from build123d import *

# Parameters (mm, degrees)
SKETCH4_R           = 3.96875
BOSS_EXTRUDE1_DEPTH = 17.5895
SKETCH5_W           = 32.258
SKETCH5_H           = 32.3469
CUT_EXTRUDE1_DEPTH  = 149.479
CUT_EXTRUDE2_REACH  = 129.277
CUT_EXTRUDE3_REACH  = 126.564
SKETCH8_R           = 4.19735
BOSS_EXTRUDE2_DEPTH = 5.4102
SKETCH9_R           = 14.8209
CUT_EXTRUDE4_DEPTH  = 102.6


with BuildPart() as part:
    # Sketch3 → Revolve1 (revolve)
    with BuildSketch(Plane.XY):
        with BuildLine():
            Line((0, 0), (22.1742, 0))
            Line((22.1742, 0), (22.1742, 6.7818))
            ThreePointArc((22.1742, 6.7818), (21.430251224, 8.577851224), (19.6342, 9.3218))
            Line((19.6342, 9.3218), (18.3134, 9.3218))
            Line((18.3134, 9.3218), (18.3134, 97.6884))
            Line((18.3134, 97.6884), (19.431, 97.6884))
            ThreePointArc((19.431, 97.6884), (21.227051224, 98.432348776), (21.971, 100.2284))
            Line((21.971, 100.2284), (21.971, 101.6))
            Line((21.971, 101.6), (0, 101.6))
            Line((0, 101.6), (0, 0))
        make_face()
    revolve(axis=Axis((0, 101.6, 0), (0, -1, 0)))

    # Sketch4 → Boss-Extrude1 (add, symmetric)
    with BuildSketch(Plane(origin=(0, 0, 0), x_dir=(0, 0, -1), z_dir=(1, 0, 0))):
        Polygon((3.319704812, 97.6884), (115.572791881, -37.744541555), (116.058945734, -61.655625383), (109.136154682, -67.393554854), (97.331039415, -71.002358659), (0, 46.427186637), align=None)
        with Locations((105.157137902, -57.289139694)):
            Circle(SKETCH4_R, mode=Mode.SUBTRACT)
    extrude(amount=BOSS_EXTRUDE1_DEPTH, both=True)

    # Sketch5 → Cut-Extrude1 (cut)
    with BuildSketch(Plane(origin=(0, -93.569618845, -77.554828616), x_dir=(1, 0, 0), z_dir=(0, -0.769917596, -0.638143319))):
        with Locations((0, -47.261148993)):
            Rectangle(SKETCH5_W, SKETCH5_H)
    extrude(amount=-CUT_EXTRUDE1_DEPTH, mode=Mode.SUBTRACT)

    # Sketch6 → Cut-Extrude2 (cut, up to next)
    with BuildSketch(Plane(origin=(0, 41.412373886, -49.963878576), x_dir=(-1, 0, 0), z_dir=(0, 0.638143319, -0.769917596)), mode=Mode.PRIVATE) as cut_extrude2_sk1:
        with BuildLine():
            Line((14.9225, -97.744891724), (14.9225, -112.907394914))
            Line((14.9225, -112.907394914), (-14.9225, -112.907394914))
            Line((-14.9225, -112.907394914), (-14.9225, -97.744891724))
            ThreePointArc((-14.9225, -97.744891724), (0, -82.822391724), (14.9225, -97.744891724))
        make_face()
    cut_extrude2_tool1 = extrude(cut_extrude2_sk1.sketch, amount=-CUT_EXTRUDE2_REACH, mode=Mode.PRIVATE) & part.part
    add(cut_extrude2_tool1.solids().sort_by_distance((0, -35.009466, -113.305835))[0], mode=Mode.SUBTRACT)

    # Sketch7 → Cut-Extrude3 (cut, up to next)
    with BuildSketch(Plane(origin=(0, 18.906399111, -22.81050181), x_dir=(1, 0, 0), z_dir=(0, -0.638143319, 0.769917596)), mode=Mode.PRIVATE) as cut_extrude3_sk1:
        with BuildLine():
            Line((-9.989016296, -117.386717047), (9.989016296, -117.386717047))
            ThreePointArc((9.989016296, -117.386717047), (0, -106.76951783), (-9.989016296, -117.386717047))
        make_face()
    cut_extrude3_tool1 = extrude(cut_extrude3_sk1.sketch, amount=-CUT_EXTRUDE3_REACH, mode=Mode.PRIVATE) & part.part
    add(cut_extrude3_tool1.solids().sort_by_distance((0, -67.984352, -94.829576))[0], mode=Mode.SUBTRACT)

    # Sketch8 → Boss-Extrude2 (add)
    with BuildSketch(Plane(origin=(17.5895, 0, 0), x_dir=(0, 0, -1), z_dir=(1, 0, 0))):
        with Locations((81.207034429, -28.363574673)):
            Circle(SKETCH8_R)
    boss_extrude2 = extrude(amount=BOSS_EXTRUDE2_DEPTH)

    # Mirror1: Boss-Extrude2 across plane
    add(boss_extrude2.mirror(Plane(origin=(0, 0, 0), x_dir=(0, 0, 1), z_dir=(1, 0, 0))))

    # Sketch9 → Cut-Extrude4 (cut, through all)
    with BuildSketch(Plane.XZ):
        Circle(SKETCH9_R)
    extrude(amount=-CUT_EXTRUDE4_DEPTH, mode=Mode.SUBTRACT)


solid = part.part
The listing builds one solid part. Answer for the finished solid, in the listing's coordinates (mm). A direction names the side the tool comes from. Give positions to 0.01 mm unless a question says otherwise; leave off trailing zeros. Write each loop counter-clockwise with the first axis right and the second up, starting at its lowest first coordinate (ties: lowest second). Pieces come first, ordered by that corner, then holes. Notation, with made-up numbers: (-10, 2) - (34, 2) arc R25 cw to (34, 15) - close; hole circle Ø1 at (2, 35.25). An arc over 180 degrees is marked (long way). One line per question, with ' | ' between items. Start each with the question number.
1. Given P1, Ø6, axis at x = 12.5, z = -86.5, coming from the +Y side; P2, Ø23.5, axis at x = 0, z = 0, coming from the +Y side; P3, Ø13.5, axis at x = -3.5, z = -10, coming from the -Y side; P4, Ø12, axis at x = -0.5, z = -34.5, coming from the +Y side, each flat-ended and moving along its own axis, determine where each tip first touches the part or whether it passes through.
2. Section C-C, the plane x = 0 is taken. Count the separate pieces of the cut face and the enclosed holes in it, then the cut area to 3 significant figures.
3. Section A-A, the plane z = 0 is taken. Determine the outline of the cut face in (x, y).
4. Straight lines are drawn through the part: line 1 (X direction, y = 46, z = -37); line 2 (Z direction, x = -9.5, y = 52); line 3 (Y direction, x = -13.5, z = -59.5). For each, find the intervals that lie inside material, in ascending order.
5. For faces 4 (the face through (-17.6, 3.44, -13.49)), 5 (the face through (-20.26, -30.92, -77.88)), 6 (the face through (-18, 9.322, -6)), determine the directions among +Z, -Z, +X, -X, +Y, -Y from which every point of the face is accessible in a straight line to the end or side of a thin tool.
6. Section D-D, the plane y = 35 is taken. Determine the outline of the cut face in (x, z), then the cut area to 3 significant figures.
7. Determine the mould class of faces 1 (the face through (14.922, -36.4, -113.5)), 2 (the face through (-16.305, -69.724, -101.512)), 3 (the face through (16.129, -7, -67)) for opening direction Z: +Z half, -Z half, draft (parallel to the pull), parting line (faces both ways), or undercut.
8. Section B-B, the plane y = 17.5 is taken. Determine the outline of the cut face in (x, z), then the cut area to 3 significant figures.
Result:
1) P1: stops at y = 0.95 | P2: passes through | P3: stops at y = 0 | P4: stops at y = 67.31
2) separate pieces: 3 | enclosed holes: 0 | area: 1,250 mm2
3) outline: (-22.17, 0) - (-14.82, 0) - (-14.82, 101.6) - (-21.97, 101.6) - (-21.97, 100.23) arc R2.54 ccw to (-19.43, 97.69) - (-18.31, 97.69) - (-18.31, 9.32) - (-19.63, 9.32) arc R2.54 ccw to (-22.17, 6.78) - close; (14.82, 0) - (22.17, 0) - (22.17, 6.78) arc R2.54 ccw to (19.63, 9.32) - (18.31, 9.32) - (18.31, 97.69) - (19.43, 97.69) arc R2.54 ccw to (21.97, 100.23) - (21.97, 101.6) - (14.82, 101.6) - close
4) line 1: x = -17.59 to -16.13, 16.13 to 17.59 | line 2: z = -41.19 to -39.29, -18.94 to -11.38, 11.38 to 15.66 | line 3: y = -25.36 to -23.07, 27.62 to 29.91
5) face 4: -Y | face 5: -X | face 6: none
6) outline: (-17.59, -55.28) - (17.59, -55.28) - (17.59, -9.47) - (15.67, -9.47) arc R18.31 ccw (long way) to (-15.67, -9.47) - (-17.59, -9.47) - close; hole (-16.13, -53.38) - (16.13, -53.38) - (16.13, -11.37) - (9.51, -11.37) arc R14.82 ccw (long way) to (-9.51, -11.37) - (-16.13, -11.37) - close | area: 469 mm2
7) face 1: draft | face 2: -Z half | face 3: undercut
8) outline: circle Ø36.63 at (0, 0); (-17.59, -69.78) - (17.59, -69.78) - (17.59, -23.98) - (-17.59, -23.98) - close; hole (-16.13, -67.89) - (16.13, -67.89) - (16.13, -25.87) - (-16.13, -25.87) - close; hole circle Ø29.64 at (0, 0) | area: 620 mm2
